```python
from build123d import *

# Parameters (mm, degrees)
SKETCH1_R               = 3.2
BOSS_EXTRUDE1_DEPTH     = 10
SKETCH2_W               = 65
SKETCH2_H               = 5
BOSS_EXTRUDE2_DEPTH     = 75
SKETCH4_R               = 3
BOSS_EXTRUDE3_DEPTH     = 3
CUT_EXTRUDE1_REACH      = 137.125
CUT_EXTRUDE1_START      = -1.8
SKETCH4_2_R             = 3
CUT_EXTRUDE2_DEPTH      = 134.324791393
CUT_EXTRUDE2_DEPTH_BACK = 134.324791393
SKETCH3_R               = 1.6
FILLET1_R               = 5
CHAMFER1_SIZE           = 10
FILLET2_R               = 1.5


with BuildPart() as part:
    # Sketch1 → Boss-Extrude1 (new body)
    with BuildSketch(Plane.XY):
        Polygon((99.5, 12.5), (87.5, 12.5), (87.5, -3), (12.5, -3), (12.5, 12.5), (0, 12.5), (0, -13), (99.5, -13), align=None)
        with Locations((93.5, 6.5)):
            Circle(SKETCH1_R, mode=Mode.SUBTRACT)
        with Locations((6.5, 6.5)):
            Circle(SKETCH1_R, mode=Mode.SUBTRACT)
    extrude(amount=BOSS_EXTRUDE1_DEPTH)

    # Sketch2 → Boss-Extrude2 (add)
    with BuildSketch(Plane.XY.offset(10)):
        with Locations((32.5, -10.5)):
            Rectangle(SKETCH2_W, SKETCH2_H)
    extrude(amount=BOSS_EXTRUDE2_DEPTH)

    # Sketch4 → Boss-Extrude3 (add)
    with BuildSketch(Plane.XZ.offset(13)):
        with Locations(Location((6.31000124, 76.457704619, 0), (0, 0, 180))):
            Circle(SKETCH4_R)
        with Locations(Location((55.31000124, 76.457704619, 0), (0, 0, 180))):
            Circle(SKETCH4_R)
        with Locations(Location((55.31000124, 18.457704619, 0), (0, 0, 180))):
            Circle(SKETCH4_R)
        with Locations(Location((6.31000124, 18.457704619, 0), (0, 0, 180))):
            Circle(SKETCH4_R)
    extrude(amount=BOSS_EXTRUDE3_DEPTH)

    # Sketch4<2> → Cut-Extrude1 (cut, up to next)
    with BuildSketch(Plane.XZ.offset(13).offset(CUT_EXTRUDE1_START), mode=Mode.PRIVATE) as cut_extrude1_sk1:
        with Locations(Location((6.31000124, 76.457704619, 0), (0, 0, 180))):
            Circle(SKETCH4_2_R)
    cut_extrude1_tool1 = extrude(cut_extrude1_sk1.sketch, amount=-CUT_EXTRUDE1_REACH, mode=Mode.PRIVATE) & part.part
    # Sketch4<2> → Cut-Extrude1 (cut, up to next)
    with BuildSketch(Plane.XZ.offset(13).offset(CUT_EXTRUDE1_START), mode=Mode.PRIVATE) as cut_extrude1_sk2:
        with Locations(Location((55.31000124, 76.457704619, 0), (0, 0, 180))):
            Circle(SKETCH4_2_R)
    cut_extrude1_tool2 = extrude(cut_extrude1_sk2.sketch, amount=-CUT_EXTRUDE1_REACH, mode=Mode.PRIVATE) & part.part
    # Sketch4<2> → Cut-Extrude1 (cut, up to next)
    with BuildSketch(Plane.XZ.offset(13).offset(CUT_EXTRUDE1_START), mode=Mode.PRIVATE) as cut_extrude1_sk3:
        with Locations(Location((55.31000124, 18.457704619, 0), (0, 0, 180))):
            Circle(SKETCH4_2_R)
    cut_extrude1_tool3 = extrude(cut_extrude1_sk3.sketch, amount=-CUT_EXTRUDE1_REACH, mode=Mode.PRIVATE) & part.part
    # Sketch4<2> → Cut-Extrude1 (cut, up to next)
    with BuildSketch(Plane.XZ.offset(13).offset(CUT_EXTRUDE1_START), mode=Mode.PRIVATE) as cut_extrude1_sk4:
        with Locations(Location((6.31000124, 18.457704619, 0), (0, 0, 180))):
            Circle(SKETCH4_2_R)
    cut_extrude1_tool4 = extrude(cut_extrude1_sk4.sketch, amount=-CUT_EXTRUDE1_REACH, mode=Mode.PRIVATE) & part.part
    add(cut_extrude1_tool1.solids().sort_by_distance((6.310001, -11.2, 76.457705))[0], mode=Mode.SUBTRACT)
    add(cut_extrude1_tool2.solids().sort_by_distance((55.310001, -11.2, 76.457705))[0], mode=Mode.SUBTRACT)
    add(cut_extrude1_tool3.solids().sort_by_distance((55.310001, -11.2, 18.457705))[0], mode=Mode.SUBTRACT)
    add(cut_extrude1_tool4.solids().sort_by_distance((6.310001, -11.2, 18.457705))[0], mode=Mode.SUBTRACT)

    # Sketch3 → Cut-Extrude2 (cut, two sides: drawn at the far end of the back side and taken through both)
    with BuildSketch(Plane.XZ.offset(13).offset(-CUT_EXTRUDE2_DEPTH_BACK)):
        with Locations((6.31000124, 76.457704619)):
            Circle(SKETCH3_R)
        with Locations((55.31000124, 76.457704619)):
            Circle(SKETCH3_R)
        with Locations((6.31000124, 18.457704619)):
            Circle(SKETCH3_R)
        with Locations((55.31000124, 18.457704619)):
            Circle(SKETCH3_R)
    extrude(amount=CUT_EXTRUDE2_DEPTH + CUT_EXTRUDE2_DEPTH_BACK, mode=Mode.SUBTRACT)

    # Fillet1
    fillet1_edges = [part.edges().sort_by_distance(p)[0] for p in [
        (32.5, -8, 10),
    ]]
    fillet(fillet1_edges, radius=FILLET1_R - 0.0001)  # a hair under: the kernel refuses the full size

    # Chamfer1
    chamfer1_edges = [part.edges().sort_by_distance(p)[0] for p in [
        (65, -8.00005, 10),
    ]]
    chamfer(chamfer1_edges, length=CHAMFER1_SIZE)

    # Fillet2
    fillet2_edges = [part.edges().sort_by_distance(p)[0] for p in [
        (9.31000124, -13, 76.457704619),
        (58.31000124, -13, 76.457704619),
        (58.31000124, -13, 18.457704619),
        (9.31000124, -13, 18.457704619),
    ]]
    fillet(fillet2_edges, radius=FILLET2_R)


solid = part.part
```
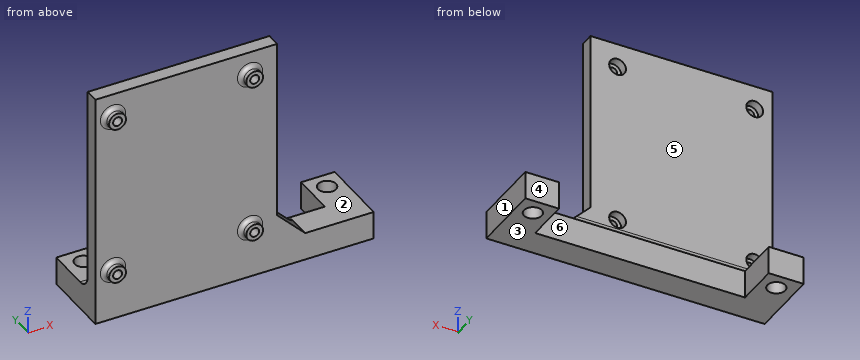
Could you check a few things on this model? Use its own coordinates, in mm. Face numbers are marked on the shaded views. A direction names the side the tool comes from. Give positions to 0.01 mm unless a question says otherwise; leave off trailing zeros. Loops run counter-clockwise (first coordinate to the right, second up) from the corner with the lowest first, then second, coordinate; pieces in that order, holes last. Notation, with made-up numbers: (31.5, -18) -> (65.5, -18) arc R31 cw to (65.5, 9) -> close; hole circle Ø1 at (37.25, -30.75). An arc over 180 degrees is marked (long way). Put each result on its own line as item: value.
(1) Imagine slicing it at D-D on y = 8.25. Write out the boundary of the cut face in (x, z), plus the area to 3 significant figures.
Computed:
outline: (0, 0) -> (3.82, 0) -> (3.82, 10) -> (0, 10) -> close; (9.18, 0) -> (12.5, 0) -> (12.5, 10) -> (9.18, 10) -> close; (87.5, 0) -> (90.82, 0) -> (90.82, 10) -> (87.5, 10) -> close; (96.18, 0) -> (99.5, 0) -> (99.5, 10) -> (96.18, 10) -> close
area: 138 mm^2
(2) Imagine slicing it at C-C on z = 8. Write out the boundary of the cut face in (x, y), plus the area to 3 significant figures.
Computed:
outline: (0, -13) -> (99.5, -13) -> (99.5, 12.5) -> (87.5, 12.5) -> (87.5, -3) -> (12.5, -3) -> (12.5, 12.5) -> (0, 12.5) -> close; hole circle Ø6.4 at (6.5, 6.5); hole circle Ø6.4 at (93.5, 6.5)
area: 1,310 mm^2
(3) Imagine slicing it at B-B on y = 2. Write out the boundary of the cut face in (x, z).
Computed:
outline: (0, 0) -> (12.5, 0) -> (12.5, 10) -> (0, 10) -> close; (87.5, 0) -> (99.5, 0) -> (99.5, 10) -> (87.5, 10) -> close
(4) Imagine slicing it at A-A on x = 93.5. Write out the boundary of the cut face in (y, z), plus the area to 3 significant figures.
Computed:
outline: (-13, 0) -> (3.3, 0) -> (3.3, 10) -> (-13, 10) -> close; (9.7, 0) -> (12.5, 0) -> (12.5, 10) -> (9.7, 10) -> close
area: 191 mm^2
(5) Thinking about a two-plate mould opening in Z: for the marked faces 1, 2 and 3, which applies, pulls with the +Z half, pulls with the -Z half, needs draft (parallel to the pull), parting line crosses it, or undercut?
Computed:
face 1: needs draft
face 2: pulls with the +Z half
face 3: pulls with the -Z half
(6) I'm going to push flat-ended pins straight in: pin 1 Ø7 at (x, z) = (6.31, 76.46) entering from +Y; pin 2 Ø12 at (x, z) = (22, 12) entering from +Y; pin 3 Ø5 at (x, z) = (22.5, 68.5) entering from -Y. Where does each tip first touch, or does it pass through?
Computed:
pin 1: y = -8
pin 2: y = -3
pin 3: y = -13
(7) Please list where these lines run through material, in increasing order: probe 1 along Z at (x, y) = (58, -8.25); probe 2 along Y at (x, z) = (89, 9.5); probe 3 along X at (y, z) = (-14.75, 17.5). Write a range as [from, to].
Computed:
probe 1: [0, 17.13], [19.79, 75.13], [77.79, 85]
probe 2: [-13, 12.5]
probe 3: [3.47, 5.03], [7.59, 9.15], [52.47, 54.03], [56.59, 58.15]
(8) For the marked faces 4, 5 and 6, which set-ups out of +Z, -Z, +X, -X, +Y, -Y let a thin tool reach every point of the face, with its end or its side?
Computed:
face 4: +Z, -Z, +X, -X, +Y
face 5: +Z, +X, -X, +Y
face 6: +Z, -Z, +Y
